Verification items for the finished model (mm, model axes). A direction names the side the tool comes from. Round coordinates to 2 decimals unless told otherwise and drop trailing zeros. Loops run counter-clockwise (first coordinate to the right, second up) from the corner with the lowest first, then second, coordinate; pieces in that order, holes last. Notation, with made-up numbers: M 33.25,69 L 61.25,69 A30 cw 61.25,104 Z; hole C 89,66.25 d2. An arc over 180 degrees is marked long. Write item = value, one per line. Start each with the question number.
from build123d import *

# Parameters (mm, degrees)
COVER_CONNECTOR_DEPTH = 210


with BuildPart() as part:
    # Sketch1 → cover_connector (new body)
    with BuildSketch(Plane.XY):
        Polygon((0, 0), (1, 0), (1, 2), (5.5, 2), (4, 3.5), (-3, 3.5), (-4.5, 2), (0, 2), align=None)
    extrude(amount=COVER_CONNECTOR_DEPTH)


solid = part.part
1. Section check A-A, the plane z = 54.5. Enter the section's corners in (x, y), and give its area (4 significant figures).
2. Gauge pin test, flat ends, axial feed: P1, Ø1, axis at x = 4, y = 2, coming from the -Z side; P2, Ø1, axis at y = 1, z = 97, coming from the +X side; P3, Ø5, axis at x = -3.5, z = 55.5, coming from the -Y side; P4, Ø1.6, axis at y = 1, z = 110.5, coming from the -X side. Record the tip position at first contact, or that the pin passes through.
3. Section check C-C, the plane y = 2.55. Enter the section's corners in (x, z).
4. Section check B-B, the plane x = -1.5. Enter the section's corners in (y, z), and give its area (3 significant figures).
5. Tool access check on faces 1 (the flat face through (0, 3, 210)), 2 (the flat face through (-2, 2, 104)), 3 (the flat face through (3, 2, 104)). Record the directions out of +Z, -Z, +X, -X, +Y, -Y that give a thin tool (end or side, any length) a straight path to the whole face; none if there is none.
6. Thickness scan on line 1 (Y direction, x = 2.75, z = 105.5); line 2 (X direction, y = 0.75, z = 59); line 3 (X direction, y = 2.25, z = 181). Record the ranges inside material, lowest first.
Computed values:
q1.outline = M -4.5,2 L 0,2 L 0,0 L 1,0 L 1,2 L 5.5,2 L 4,3.5 L -3,3.5 Z
q1.area = 14.75 mm2
q2.P1 = 0
q2.P2 = 1
q2.P3 = 2
q2.P4 = 0
q3.outline = M -3.95,0 L 4.95,0 L 4.95,210 L -3.95,210 Z
q4.outline = M 2,0 L 3.5,0 L 3.5,210 L 2,210 Z
q4.area = 315 mm2
q5.face_1 = +Z, +X, -X, +Y, -Y
q5.face_2 = +Z, -Z, -X, -Y
q5.face_3 = +Z, -Z, +X, -Y
q6.line_1 = 2 to 3.5
q6.line_2 = 0 to 1
q6.line_3 = -4.25 to 5.25
